from build123d import *

# Parameters (mm, degrees)
BACK_PLATE_MAIN_R          = 101.6
BOSS_EXTRUDE1_DEPTH        = 6.35
F_9_0_196_DIAMETER_HOLE1_D = 4.9784
CLEARANCE_CUTOUT_R         = 25.4
CUT_EXTRUDE1_DEPTH         = 3.81


with BuildPart() as part:
    # Back Plate Main → Boss-Extrude1 (new body)
    with BuildSketch(Plane(origin=(0, 0, 0), x_dir=(1, 0, 0), z_dir=(0, 1, 0))):
        with Locations(Location((0, 0, 0), (0, 0, 270))):
            Circle(BACK_PLATE_MAIN_R)
    extrude(amount=-BOSS_EXTRUDE1_DEPTH)

    # #9 (0.196) Diameter Hole1 (through all)
    with Locations(Plane(origin=(0, 0, 0), x_dir=(1, 0, 0), z_dir=(0, 1, 0))):
        with Locations((0, 95.25), (82.48891971, 47.625), (82.48891971, -47.625), (0, -95.25), (-82.48891971, -47.625), (-82.48891971, 47.625), (-72.965733207, 61.225519823), (16.539988923, 93.802938474), (89.50572213, 32.577418652), (72.965733207, -61.225519823), (-16.539988923, -93.802938474), (-89.50572213, -32.577418652)):
            Hole(F_9_0_196_DIAMETER_HOLE1_D / 2)

    # Clearance Cutout → Cut-Extrude1 (cut)
    with BuildSketch(Plane.XZ.offset(6.35)):
        with Locations(Location((0, 0, 0), (0, 0, 270))):
            Circle(CLEARANCE_CUTOUT_R)
    extrude(amount=-CUT_EXTRUDE1_DEPTH, mode=Mode.SUBTRACT)


solid = part.part
Input: part model. Units: mm. Frame: model coordinates. A direction names the side the tool comes from. Give positions to 0.01 mm unless a question says otherwise; leave off trailing zeros. Order: outer loops, then holes, each group sorted by start corner. A loop starts at its lowest first (then second) coordinate and runs counter-clockwise, first axis right, second up.
Q1. Section B-B on z = 0. Output: boundary loops of the cut face in (x, y), and give its area (3 significant figures).
Checked values:
outline: (-101.6, -6.35) - (-25.4, -6.35) - (-25.4, -2.54) - (25.4, -2.54) - (25.4, -6.35) - (101.6, -6.35) - (101.6, 0) - (-101.6, 0) - close
area: 1,100 mm2
Q2. Section A-A on x = 0. Output: boundary loops of the cut face in (y, z).
Checked values:
outline: (-6.35, -101.6) - (0, -101.6) - (0, -97.74) - (-6.35, -97.74) - close; (-6.35, -92.76) - (0, -92.76) - (0, 92.76) - (-6.35, 92.76) - (-6.35, 25.4) - (-2.54, 25.4) - (-2.54, -25.4) - (-6.35, -25.4) - close; (-6.35, 97.74) - (0, 97.74) - (0, 101.6) - (-6.35, 101.6) - close
Q3. Contact query for a flat-ended pin moving along its axis: pin 1 Ø15 at (x, z) = (0, -9) entering from -Y. Output: stop coordinate, or through.
Checked values:
pin 1: stops at y = -2.54
Q4. Section C-C on y = -3.5. State how many separate pieces and enclosed holes the cut face has, and give its area (3 significant figures).
Checked values:
separate pieces: 1
enclosed holes: 13
area: 30,200 mm2
Q5. Section D-D on x = -68. Output: boundary loops of the cut face in (y, z), and give its area (3 significant figures).
Checked values:
outline: (-6.35, -75.49) - (0, -75.49) - (0, 75.49) - (-6.35, 75.49) - close
area: 959 mm2
Q6. Ray query, probe 1 along Z at (x, y) = (-15, -5); probe 2 along X at (y, z) = (-4, -59.5); probe 3 along X at (y, z) = (-4.75, 19). Return the intervals inside material, ascending.
Checked values:
probe 1: z = -100.49 to -20.5, 20.5 to 91.85, 95.76 to 100.49
probe 2: x = -82.35 to -74.76, -71.17 to 82.35
probe 3: x = -99.81 to -16.86, 16.86 to 99.81
Q7. Set-up query: faces 4 (the cylindrical face through (-15.456, -4.472, 20.157)), 5 (the cylindrical face through (-80, -3.22, 47.52)). Return all of +Z, -Z, +X, -X, +Y, -Y with unobstructed straight access to the full face (end or side cutting, diameter ignored); none if empty.
Checked values:
face 4: -Y
face 5: +Y, -Y
Q8. Draft query along Z for faces 1 (the cylindrical face through (-61.82, -3.13, -80.63)), 2 (the cylindrical face through (70.59, -3.22, 60.48)), 3 (the flat face through (-21, -6.35, 21)). Return one class per face: +Z half, -Z half, draft (parallel to the pull), parting line (faces both ways), or undercut.
Checked values:
face 1: parting line
face 2: undercut
face 3: draft
